Here's how the part is built. I have some questions about the finished solid (model axes, mm). Coordinates: 2 decimals unless noted, no trailing zeros. Loops run counter-clockwise (first coordinate to the right, second up) from the corner with the lowest first, then second, coordinate; pieces in that order, holes last. Notation, with made-up numbers: (-5, -5.5) -> (2, -5.5) arc R11 cw to (2, 15.5) -> close; hole circle Ø1 at (43, -21.75). An arc over 180 degrees is marked (long way). Answer as a JSON object with one key per item and string values. Group by question number.
Q1. I'm going to push flat-ended pins straight in: pin 1 (8 mm diameter, centred on x = 27, z = 9.5, fed in from -Y); pin 2 (2 mm diameter, centred on x = 30.5, z = -117, fed in from -Y); pin 3 (4 mm diameter, centred on y = -25, z = -95.5, fed in from +X). Where does each tip first touch, or does it pass through?
Q2. I want a section at C-C on z = -111. Write out the boundary of the cut face in (x, y), then the cut area to 3 significant figures.
Q3. Thinking about a two-plate mould opening in X: for faces 1 (the cylindrical face through (0.15, -60.23, -70.08)), 2 (the flat face through (0, -58, 28.369)), 3 (the cylindrical face through (-1.396, -63.485, -61.776)), which applies, released by +X, released by -X, zero draft, split by the parting line, or undercut?
Q4. I want a section at D-D on y = -31. Write out the boundary of the cut face in (x, z), then the cut area to 3 significant figures.
Q5. I want a section at B-B on y = -48.5. Write out the boundary of the cut face in (x, z).
Q6. I need wall thicknesses on line 1 (Z direction, x = 0, y = -60); line 2 (X direction, y = -10, z = -61); line 3 (X direction, y = -17, z = -71.5). Which ranges of each line are inside material? Lowest first, please.
Q7. I want a section at A-A on x = 0. Write out the boundary of the cut face in (y, z).
```python
from build123d import *

# Parameters (mm, degrees)
SKETCH2_W          = 177.8
SKETCH2_H          = 6.35
REVOLVE1_ANGLE     = 180
SKETCH3_R          = 3.327499949
CUT_EXTRUDE1_DEPTH = 175.339362144


with BuildPart() as part:
    # Sketch2 → Revolve1 (revolve)
    with BuildSketch(Plane(origin=(0, 0, 0), x_dir=(0, 0, -1), z_dir=(0, -1, 0))):
        with Locations((60.53129924, -60.325)):
            Rectangle(SKETCH2_W, SKETCH2_H)
    revolve(axis=Axis((0, 0, 0), (0, 0, 1)), revolution_arc=REVOLVE1_ANGLE)

    # Sketch3 → Cut-Extrude1 (cut, through all)
    with BuildSketch(Plane(origin=(0, 0, 0), x_dir=(1, 0, 0), z_dir=(0, 1, 0))):
        with Locations(Location((0, 66.75429924, 0), (0, 0, 270))):
            Circle(SKETCH3_R)
        with Locations(Location((0, 54.30829924, 0), (0, 0, 270))):
            Circle(SKETCH3_R)
    extrude(amount=-CUT_EXTRUDE1_DEPTH, mode=Mode.SUBTRACT)


solid = part.part
```
Result set:
{
 "1": {"pin 1": "stops at y = -59.19", "pin 2": "stops at y = -56.23", "pin 3": "stops at x = 59.19"},
 "2": {"outline": "(-63.5, 0) arc R63.5 ccw to (63.5, 0) -> (57.15, 0) arc R57.15 cw to (-57.15, 0) -> close", "area": "1,200 mm²"},
 "3": {"face 1": "undercut", "face 2": "zero draft", "face 3": "split by the parting line"},
 "4": {"outline": "(-55.42, -149.43) -> (-48.01, -149.43) -> (-48.01, 28.37) -> (-55.42, 28.37) -> close; (48.01, -149.43) -> (55.42, -149.43) -> (55.42, 28.37) -> (48.01, 28.37) -> close", "area": "2,630 mm²"},
 "5": {"outline": "(-40.99, -149.43) -> (-30.23, -149.43) -> (-30.23, 28.37) -> (-40.99, 28.37) -> close; (30.23, -149.43) -> (40.99, -149.43) -> (40.99, 28.37) -> (30.23, 28.37) -> close"},
 "6": {"line 1": "z = -149.43 to -70.08, -63.43 to -57.64, -50.98 to 28.37", "line 2": "x = -62.71 to -56.27, 56.27 to 62.71", "line 3": "x = -61.18 to -54.56, 54.56 to 61.18"},
 "7": {"outline": "(-63.5, -149.43) -> (-57.15, -149.43) -> (-57.15, -70.08) -> (-63.5, -70.08) -> close; (-63.5, -63.43) -> (-57.15, -63.43) -> (-57.15, -57.64) -> (-63.5, -57.64) -> close; (-63.5, -50.98) -> (-57.15, -50.98) -> (-57.15, 28.37) -> (-63.5, 28.37) -> close"}
}
